Build history of the part. All positions in model axes, mm. Face numbers are marked on the shaded views. A direction names the side the tool comes from. Give positions to 0.01 mm unless a question says otherwise; leave off trailing zeros. Loops run counter-clockwise (first coordinate to the right, second up) from the corner with the lowest first, then second, coordinate; pieces in that order, holes last.
1) Band-saw the part on B-B on z = 1. List the corners of the cut face in (x, y).
2) Two-plate mould, pull along Y, no slides. Class the marked faces 1, 2 and 3: +Y half, -Y half, draft (parallel to the pull), parting line (faces both ways), or undercut.
3) Flat gauge pins, fed straight in: P1, Ø4, axis at x = -18.5, z = 7, coming from the +Y side; P2, Ø0.9, axis at y = 29, z = 10, coming from the -X side; P3, Ø8, axis at x = -63, y = 26, coming from the +Z side; P4, Ø6, axis at x = -36, z = 7.5, coming from the -Y side. Where does each tip first touch, or does it go through?
4) Wall check: line 1 (X direction, y = 14.5, z = 5.25); line 2 (Z direction, x = -42, y = 25.5); line 3 (Y direction, x = -33, z = 3.5). Give the ranges that are in metal, low to high.
5) 3-axis set-ups, long thin cutter, end or side, ignore diameter. For the marked faces 4, 5 and 6: which of +Z, -Z, +X, -X, +Y, -Y reach the whole face in a straight line?
6) Band-saw the part on C-C on y = 20. List the corners of the cut face in (x, z), then the cut area to 3 significant figures.
7) Band-saw the part on A-A on x = -45. List the corners of the cut face in (y, z).
8) Band-saw the part on D-D on x = -25. List the corners of the cut face in (y, z), then the cut area to 3 significant figures.
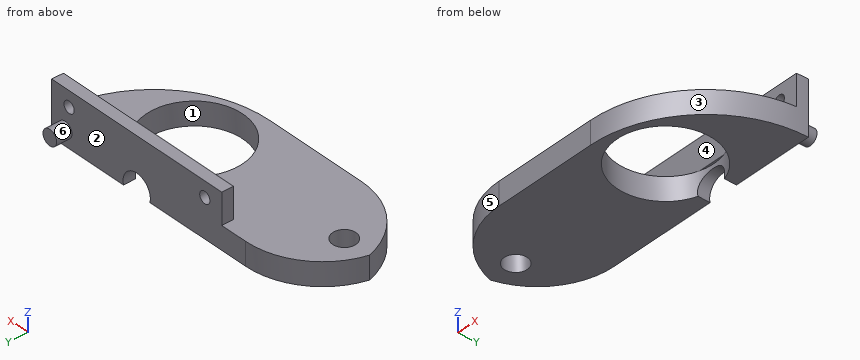
```python
from build123d import *

# Parameters (mm, degrees)
ESQUISSE1_W                  = 77
ESQUISSE1_H                  = 30
BOSS_EXTRU_1_DEPTH           = 6
ESQUISSE2_R                  = 12.5
ESQUISSE2_R_2                = 3
ENL_V_MAT_EXTRU_1_DEPTH      = 6
ESQUISSE3_W                  = 50
ESQUISSE3_H                  = 3
BOSS_EXTRU_2_DEPTH           = 8
ENL_V_MAT_EXTRU_2_REACH      = 85.815
ENL_V_MAT_EXTRU_2_END_RADIUS = 12.5
ESQUISSE5_R                  = 4
CONG_1_R                     = 20
CONG_2_R                     = 30
ESQUISSE6_R                  = 2
BOSS_EXTRU_3_DEPTH           = 4
ESQUISSE7_R                  = 1.5
ENL_V_MAT_EXTRU_3_DEPTH      = 10


with BuildPart() as part:
    # Esquisse1 → Boss.-Extru.1 (new body)
    with BuildSketch(Plane.XY):
        with Locations((-38.5, 15)):
            Rectangle(ESQUISSE1_W, ESQUISSE1_H)
    extrude(amount=BOSS_EXTRU_1_DEPTH)

    # Esquisse2 → Enlèv. mat.-Extru.1 (cut)
    with BuildSketch(Plane.XY.offset(6)):
        with Locations((-25, 15)):
            Circle(ESQUISSE2_R)
        with Locations((-69, 15)):
            Circle(ESQUISSE2_R_2)
    extrude(amount=-ENL_V_MAT_EXTRU_1_DEPTH, mode=Mode.SUBTRACT)

    # Esquisse3 → Boss.-Extru.2 (add)
    with BuildSketch(Plane.XY.offset(6)):
        with Locations((-25, 28.5)):
            Rectangle(ESQUISSE3_W, ESQUISSE3_H)
    extrude(amount=BOSS_EXTRU_2_DEPTH)

    # Enlèv. mat.-Extru.2: up to this cylinder (the profile starts outside it)
    enl_v_mat_extru_2_end = Plane(origin=(-25, 15, 1), z_dir=(0, 0, 1)) * Cylinder(ENL_V_MAT_EXTRU_2_END_RADIUS, 197.63, mode=Mode.PRIVATE)
    # Esquisse5 → Enlèv. mat.-Extru.2 (cut, up to the surface)
    with BuildSketch(Plane(origin=(0, 30, 0), x_dir=(1, 0, 0), z_dir=(0, 1, 0)), mode=Mode.PRIVATE) as enl_v_mat_extru_2_sk1:
        with Locations((-25, -1)):
            Circle(ESQUISSE5_R)
    enl_v_mat_extru_2_tool1 = extrude(enl_v_mat_extru_2_sk1.sketch, amount=-ENL_V_MAT_EXTRU_2_REACH, mode=Mode.PRIVATE) - enl_v_mat_extru_2_end
    add(enl_v_mat_extru_2_tool1.solids().sort_by_distance((-25, 30, 1))[0], mode=Mode.SUBTRACT)

    # Congé1
    # the kernel refuses this fillet: 20 mm, written as the material it takes off along each edge
    with BuildSketch(Plane(origin=(-77, 30, -50), x_dir=(1, 0, 0), z_dir=(0, 0, 1))) as cong_1_piece_1:
        with BuildLine():
            CenterArc((CONG_1_R, -CONG_1_R), CONG_1_R, 90, 90)
            Line((0, -CONG_1_R), (0, 0))
            Line((0, 0), (CONG_1_R, 0))
        make_face()
    extrude(amount=106, mode=Mode.SUBTRACT)
    with BuildSketch(Plane(origin=(-77, 0, -50), x_dir=(1, 0, 0), z_dir=(0, 0, 1))) as cong_1_piece_2:
        with BuildLine():
            CenterArc((CONG_1_R, CONG_1_R), CONG_1_R, 180, 90)
            Line((0, CONG_1_R), (0, 0))
            Line((0, 0), (CONG_1_R, 0))
        make_face()
    extrude(amount=106, mode=Mode.SUBTRACT)

    # Congé2
    # the kernel refuses this fillet: 30 mm, written as the material it takes off along each edge
    with BuildSketch(Plane(origin=(0, 0, -75), x_dir=(-1, 0, 0), z_dir=(0, 0, 1))) as cong_2_piece_1:
        with BuildLine():
            CenterArc((CONG_2_R, -CONG_2_R), CONG_2_R, 90, 90)
            Line((0, -CONG_2_R), (0, 0))
            Line((0, 0), (CONG_2_R, 0))
        make_face()
    extrude(amount=156, mode=Mode.SUBTRACT)

    # Esquisse6 → Boss.-Extru.3 (add)
    with BuildSketch(Plane(origin=(0, 30, 0), x_dir=(1, 0, 0), z_dir=(0, 1, 0))):
        with Locations((-4, -4)):
            Circle(ESQUISSE6_R)
    extrude(amount=BOSS_EXTRU_3_DEPTH)

    # Esquisse7 → Enlèv. mat.-Extru.3 (cut)
    with BuildSketch(Plane.XZ.offset(-27)):
        with Locations((-45, 10)):
            Circle(ESQUISSE7_R)
        with Locations((-5.150376887, 10)):
            Circle(ESQUISSE7_R)
    extrude(amount=-ENL_V_MAT_EXTRU_3_DEPTH, mode=Mode.SUBTRACT)


solid = part.part
```
Findings below:
1. outline: (-76.36, 15) arc R20 ccw to (-57, 0) - (-30, 0) arc R30 ccw to (0, 30) - (-21, 30) - (-21, 26.84) arc R12.5 cw (long way) to (-29, 26.84) - (-29, 30) - (-57, 30) arc R20 ccw to start; hole circle Ø6 at (-69, 15)
2. face 1: undercut
2. face 2: +Y half
2. face 3: -Y half
3. P1: stops at y = 30
3. P2: stops at x = -50
3. P3: stops at z = 6
3. P4: stops at y = 0
4. line 1: x = -76.23 to -71.96, -66.04 to -37.49, -12.51 to -4.31
4. line 2: z = 0 to 6
4. line 3: y = 0 to 5.4, 24.6 to 30
5. face 4: +Z, +X, -X, -Y
5. face 5: +Z, -Z, -X, -Y
5. face 6: +Y
6. outline: (-74.32, 0) - (-36.46, 0) - (-36.46, 6) - (-74.32, 6) - close; (-13.54, 0) - (-1.72, 0) - (-1.72, 6) - (-13.54, 6) - close
6. area: 298 mm2
7. outline: (0, 0) - (30, 0) - (30, 8.5) - (27, 8.5) - (27, 6) - (0, 6) - close; (27, 11.5) - (30, 11.5) - (30, 14) - (27, 14) - close
8. outline: (0.42, 0) - (2.5, 0) - (2.5, 6) - (0.42, 6) - close; (27, 6) - (27.5, 6) - (27.5, 5) - (30, 5) - (30, 14) - (27, 14) - close
8. area: 39.0 mm2
